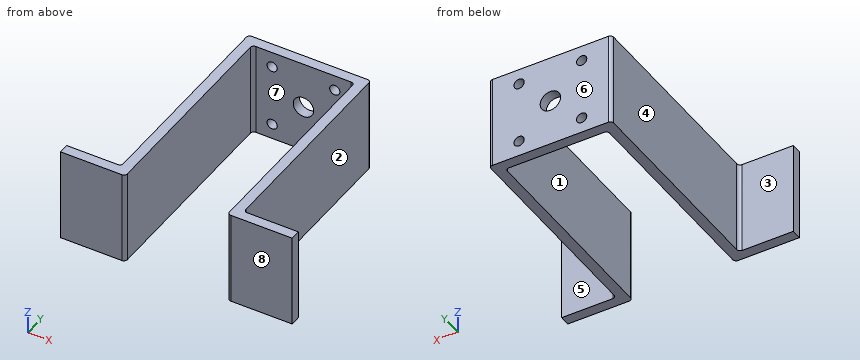
from build123d import *

# Parameters (mm, degrees)
BOSS_EXTRUDE1_DEPTH = 13.75
SKETCH2_R           = 3
SKETCH2_R_2         = 1.5
CUT_EXTRUDE1_DEPTH  = 66


with BuildPart() as part:
    # Sketch1 → Boss-Extrude1 (new body, symmetric)
    with BuildSketch(Plane.XY):
        with BuildLine():
            Line((0, 37.295033495), (-14, 37.295033495))
            ThreePointArc((-14, 37.295033495), (-14.707106781, 37.002140277), (-15, 36.295033495))
            Line((-15, 36.295033495), (-15, -23.704966505))
            ThreePointArc((-15, -23.704966505), (-15.292893219, -24.412073286), (-16, -24.704966505))
            Line((-16, -24.704966505), (-34, -24.704966505))
            Line((-34, -24.704966505), (-34, -21.704966505))
            Line((-34, -21.704966505), (-19, -21.704966505))
            ThreePointArc((-19, -21.704966505), (-18.292893219, -21.412073286), (-18, -20.704966505))
            Line((-18, -20.704966505), (-18, 39.295033495))
            ThreePointArc((-18, 39.295033495), (-17.707106781, 40.002140277), (-17, 40.295033495))
            Line((-17, 40.295033495), (0, 40.295033495))
            Line((0, 40.295033495), (0, 37.295033495))
        make_face()
    boss_extrude1 = extrude(amount=BOSS_EXTRUDE1_DEPTH, both=True)

    # Mirror1: Boss-Extrude1 across plane
    add(boss_extrude1.mirror(Plane(origin=(0, 0, 0), x_dir=(0, 0, 1), z_dir=(1, 0, 0))))

    # Sketch2 → Cut-Extrude1 (cut, through all)
    with BuildSketch(Plane(origin=(0, 40.295033495, 0), x_dir=(1, 0, 0), z_dir=(0, 1, 0))):
        Circle(SKETCH2_R)
        with Locations((-9.19, 9.19)):
            Circle(SKETCH2_R_2)
        with Locations((9.19, 9.19)):
            Circle(SKETCH2_R_2)
        with Locations((9.19, -9.19)):
            Circle(SKETCH2_R_2)
        with Locations((-9.19, -9.19)):
            Circle(SKETCH2_R_2)
    extrude(amount=-CUT_EXTRUDE1_DEPTH, mode=Mode.SUBTRACT)


solid = part.part
The model under review builds one solid part; all positions refer to its coordinate system, in mm. Face numbers are marked on the shaded views. A direction names the side the tool comes from. Round coordinates to 2 decimals unless told otherwise and drop trailing zeros. Loops run counter-clockwise (first coordinate to the right, second up) from the corner with the lowest first, then second, coordinate; pieces in that order, holes last. Notation, with made-up numbers: (13.5, 2.25) - (57.5, 2.25) arc R17 ccw to (57.5, 19.25) - close; hole circle Ø2 at (-25, 77.5). An arc over 180 degrees is marked (long way). Use CSV: the item, a comma, the result in double quotes.
(1) Take a section at C-C, the plane z = -9.19. Give the boundary of the cut face in (x, y), plus the area to 3 significant figures.
Working result:
outline,"(-34, -24.7) - (-16, -24.7) arc R1 ccw to (-15, -23.7) - (-15, 36.3) arc R1 cw to (-14, 37.3) - (-10.69, 37.3) - (-10.69, 40.3) - (-17, 40.3) arc R1 ccw to (-18, 39.3) - (-18, -20.7) arc R1 cw to (-19, -21.7) - (-34, -21.7) - close; (-7.69, 37.3) - (7.69, 37.3) - (7.69, 40.3) - (-7.69, 40.3) - close; (10.69, 37.3) - (14, 37.3) arc R1 cw to (15, 36.3) - (15, -23.7) arc R1 ccw to (16, -24.7) - (34, -24.7) - (34, -21.7) - (19, -21.7) arc R1 cw to (18, -20.7) - (18, 39.3) arc R1 ccw to (17, 40.3) - (10.69, 40.3) - close"
area,"558 mm^2"
(2) For line 1 (Z direction, x = 9, y = 38); line 2 (X direction, y = 38.7, z = -9.19); line 3 (X direction, y = -8, z = 0), list the stretches that pass through material, from the lowest coordinate up.
Working result:
line 1,"z = -13.75 to -10.68, -7.7 to 7.7, 10.68 to 13.75"
line 2,"x = -18 to -10.69, -7.69 to 7.69, 10.69 to 18"
line 3,"x = -18 to -15, 15 to 18"
(3) Clearance check with flat-ended pins moving along their axes: P1, Ø5, axis at x = 9.19, z = -9.19, coming from the +Y side; P2, Ø8, axis at x = -5, z = 0.5, coming from the -Y side; P3, Ø3, axis at y = 17.5, z = 10, coming from the +X side; P4, Ø8, axis at y = -6.5, z = -5, coming from the -X side. State where each tip first meets the part, or that it passes through.
Working result:
P1,"stops at y = 40.3"
P2,"stops at y = 37.3"
P3,"stops at x = 18"
P4,"stops at x = -18"
(4) The part is to be moulded in two halves that separate along X. For the marked faces 1, 2 and 3, say which applies: pulls with the +X half, pulls with the -X half, needs draft (parallel to the pull), parting line crosses it, or undercut.
Working result:
face 1,"undercut"
face 2,"pulls with the +X half"
face 3,"needs draft"
(5) Machinability: for the marked faces 4, 5, 6, 7 and 8, which of the approach directions +Z, -Z, +X, -X, +Y, -Y give a long, thin tool a straight path to every point of the face, cutting with its end or side? Answer none if there is none.
Working result:
face 4,"+Z, -Z, -X, +Y"
face 5,"+Z, -Z, +X, +Y"
face 6,"+Z, -Z, +X, -X, +Y"
face 7,"+Z, -Z, -Y"
face 8,"+Z, -Z, +X, -X, -Y"
(6) Take a section at B-B, the plane y = 25. Give the boundary of the cut face in (x, z).
Working result:
outline,"(-18, -13.75) - (-15, -13.75) - (-15, 13.75) - (-18, 13.75) - close; (15, -13.75) - (18, -13.75) - (18, 13.75) - (15, 13.75) - close"
(7) Take a section at A-A, the plane x = 0. Give the boundary of the cut face in (y, z).
Working result:
outline,"(37.3, -13.75) - (40.3, -13.75) - (40.3, -3) - (37.3, -3) - close; (37.3, 3) - (40.3, 3) - (40.3, 13.75) - (37.3, 13.75) - close"
(8) Take a section at D-D, the plane x = -9.19. Give the boundary of the cut face in (y, z).
Working result:
outline,"(37.3, -13.75) - (40.3, -13.75) - (40.3, -10.69) - (37.3, -10.69) - close; (37.3, -7.69) - (40.3, -7.69) - (40.3, 7.69) - (37.3, 7.69) - close; (37.3, 10.69) - (40.3, 10.69) - (40.3, 13.75) - (37.3, 13.75) - close"
